Verification items for this drawing (mm, ordinates from the low corner). Round coordinates to 2 decimals unless told otherwise and drop trailing zeros. Write each loop counter-clockwise with the first axis right and the second up, starting at its lowest first coordinate (ties: lowest second). Pieces come first, ordered by that corner, then holes. Notation, with made-up numbers: (-21, 84) -> (25, 84) arc R14 ccw to (25, 101) -> close; hole circle Ø2 at (0.25, 9.5). An arc over 180 degrees is marked (long way). Return JSON: item names as keys, results as strings. Group by question number.
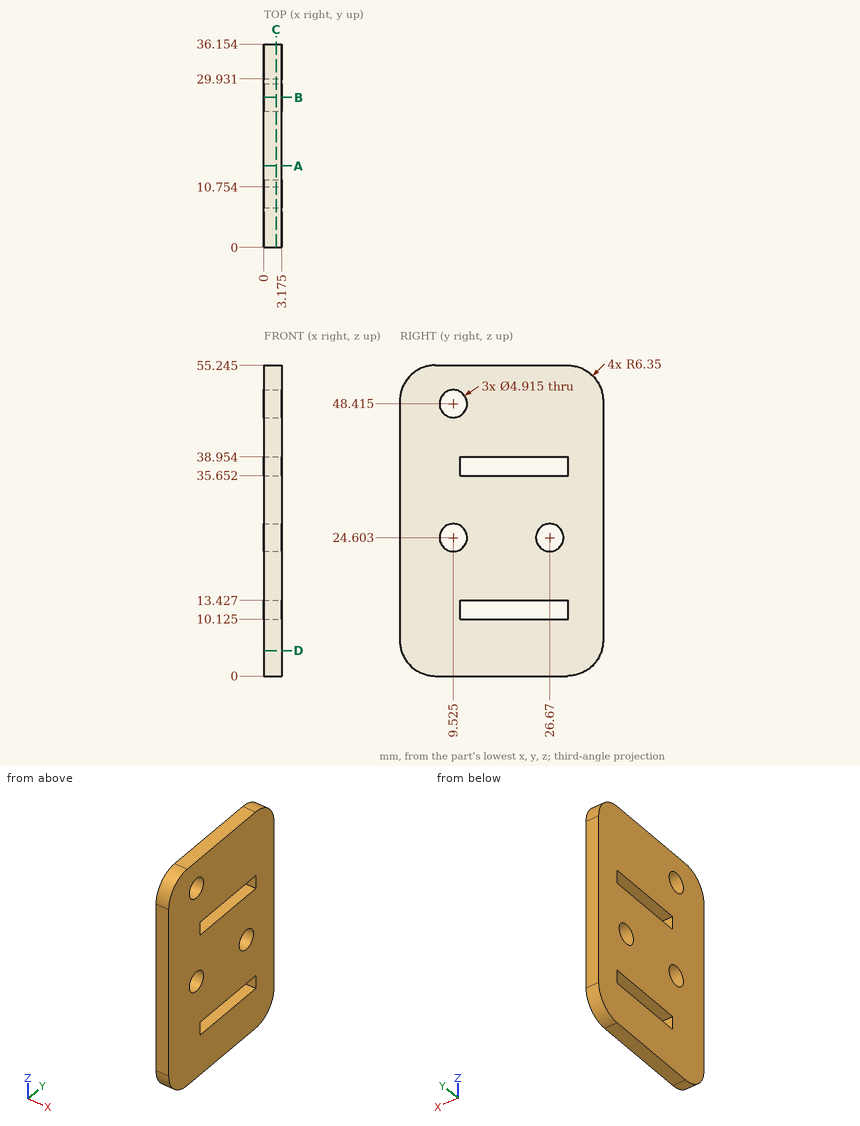
1) Material ranges on probe 1 along Y at (x, z) = (0.7, 24.5) (1 decimal); probe 2 along Y at (x, z) = (1.1, 36) (1 decimal); probe 3 along Z at (x, y) = (1.65, 19) (1 decimal), recorded low to high. Write a range as [from, to].
2) Sectioned sample at A-A on y = 14.5. Enter the section's corners in (x, z) (1 decimal).
3) Sectioned sample at D-D on z = 4.5. Enter the section's corners in (x, y) (1 decimal), and give its area (3 significant figures).
4) Sectioned sample at C-C on x = 2.15. State how many separate pieces and enclosed holes the cut face has, and give its area (3 significant figures).
5) Sectioned sample at B-B on y = 26.67. Enter the section's corners in (x, z) (1 decimal), and give its area (3 significant figures).
6) Go/stop test with a flat-tipped pin: P1, Ø4.5, axis at y = 9.53, z = 24.6, coming from the +X side. Record where the tip stops, or that it passes through.
Evaluation:
{
 "1": {"probe 1": "y = [0, 7.1], [12, 24.2], [29.1, 36.2]", "probe 2": "y = [0, 10.8], [29.9, 36.2]", "probe 3": "z = [0, 10.1], [13.4, 35.7], [39, 55.2]"},
 "2": {"outline": "(0, 0) -> (3.2, 0) -> (3.2, 10.1) -> (0, 10.1) -> close; (0, 13.4) -> (3.2, 13.4) -> (3.2, 35.7) -> (0, 35.7) -> close; (0, 39) -> (3.2, 39) -> (3.2, 55.2) -> (0, 55.2) -> close"},
 "3": {"outline": "(0, 0.3) -> (3.2, 0.3) -> (3.2, 35.9) -> (0, 35.9) -> close", "area": "113 mm2"},
 "4": {"separate pieces": "1", "enclosed holes": "5", "area": "1,780 mm2"},
 "5": {"outline": "(0, 0) -> (3.2, 0) -> (3.2, 10.1) -> (0, 10.1) -> close; (0, 13.4) -> (3.2, 13.4) -> (3.2, 22.1) -> (0, 22.1) -> close; (0, 27.1) -> (3.2, 27.1) -> (3.2, 35.7) -> (0, 35.7) -> close; (0, 39) -> (3.2, 39) -> (3.2, 55.2) -> (0, 55.2) -> close", "area": "139 mm2"},
 "6": {"P1": "passes through"}
}
